```python
from build123d import *

# Parameters (mm, degrees)
EXTRUDE_THIN1_DEPTH = 206.375
FILLET1_R           = 0.889


with BuildPart() as part:
    # Sketch1 → Extrude-Thin1 (new body)
    with BuildSketch(Plane.XY):
        with BuildLine():
            Line((-0.79375, 3.074180531), (0, 0))
            ThreePointArc((0, 0), (-9.091384352, 4.706963909), (-12.7, 14.2875))
            Line((-12.7, 14.2875), (-1.285875, 14.2875))
            Line((-1.285875, 14.2875), (-0.889, 20.625085521))
            Line((-0.889, 20.625085521), (-0.001738027, 20.569523021))
            Line((-0.001738027, 20.569523021), (-0.450804908, 13.3985))
            Line((-0.450804908, 13.3985), (-11.787335474, 13.3985))
            ThreePointArc((-11.787335474, 13.3985), (-8.569392416, 5.460475486), (-1.20057239, 1.093796873))
            Line((-1.20057239, 1.093796873), (-1.654520549, 2.851930531))
            Line((-1.654520549, 2.851930531), (-0.79375, 3.074180531))
        make_face()
    extrude(amount=-EXTRUDE_THIN1_DEPTH)

    # Fillet1
    fillet1_edges = [part.edges().sort_by_distance(p)[0] for p in [
        (-0.450804908, 13.3985, -103.1875),
        (-12.7, 14.2875, -103.1875),
    ]]
    fillet(fillet1_edges, radius=FILLET1_R)


solid = part.part
```
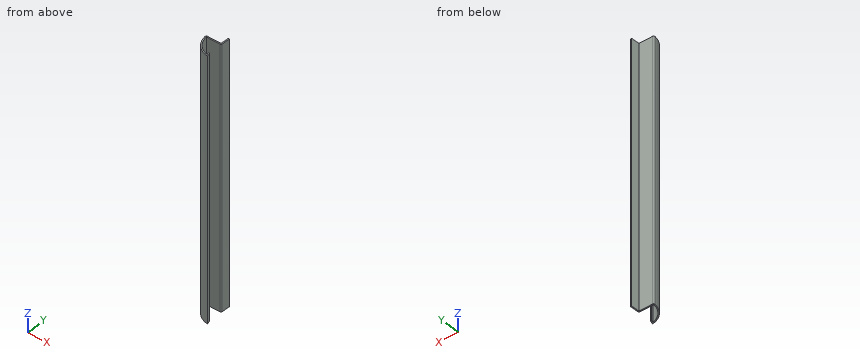
The model under review builds one solid part; all positions refer to its coordinate system, in mm. Round coordinates to 2 decimals unless told otherwise and drop trailing zeros. Loops run counter-clockwise (first coordinate to the right, second up) from the corner with the lowest first, then second, coordinate; pieces in that order, holes last. Notation, with made-up numbers: M 48,-16 L 54,-16 A14 cw 54,-4 Z; hole C 55.25,22.25 d6. An arc over 180 degrees is marked long. Put each result on its own line as item: value.
Q1. To check wall thickness, follow L1, parallel to Y at x = -8.5, z = -190.5; L2, parallel to Y at x = -4.75, z = -44.5; L3, parallel to X at y = 2.5, z = -37. State the ranges of each line that lie inside material, in increasing order.
Result set:
L1: y = 4.08 to 5.38, 13.4 to 14.29
L2: y = 1.39 to 2.39, 13.4 to 14.29
L3: x = -6.61 to -4.94, -1.56 to -0.65
Q2. Consider section B-B, the plane x = -8.25. Give the boundary of the cut face in (y, z) (1 decimal).
Result set:
outline: M 3.8,-206.4 L 5.1,-206.4 L 5.1,0 L 3.8,0 Z; M 13.4,-206.4 L 14.3,-206.4 L 14.3,0 L 13.4,0 Z
Q3. For pin 1 (5.5 mm diameter, centred on x = -6.5, z = -107.5, fed in from +Y); pin 2 (1.5 mm diameter, centred on y = 10.5, z = -54, fed in from -X); pin 3 (4 mm diameter, centred on x = -6.5, z = -136.5, fed in from -Y); pin 4 (6 mm diameter, centred on x = -3.5, y = 8.5, fed in from +Z), all flat-tipped, find the tip position at first contact; note any pin that passes through.
Result set:
pin 1: stops at y = 14.29
pin 2: stops at x = -12.39
pin 3: stops at y = 1.27
pin 4: passes through
Q4. Consider section A-A, the plane z = -161.5. Give the boundary of the cut face in (x, y) (1 decimal), then the cut area to 3 significant figures.
Result set:
outline: M -12.7,13.3 A14.3 ccw 0,0 L -0.8,3.1 L -1.7,2.9 L -1.2,1.1 A13.4 cw -11.8,13.4 L -1.3,13.4 A0.9 ccw -0.4,14.2 L 0,20.6 L -0.9,20.6 L -1.3,14.3 L -11.8,14.3 A0.9 ccw Z
area: 35.1 mm²
Q5. Consider section C-C, the plane y = 8.5. Give the boundary of the cut face in (x, z) (3 decimals).
Result set:
outline: M -11.514,-206.375 L -10.539,-206.375 L -10.539,0 L -11.514,0 Z
Q6. Consider section D-D, the plane y = 18.25. Give the boundary of the cut face in (x, z) (3 decimals).
Result set:
outline: M -1.038,-206.375 L -0.147,-206.375 L -0.147,0 L -1.038,0 Z
